Source: CAD feature listing. Evaluate the final solid. Frame: model axes, mm. Face numbers are marked on the shaded views. A direction names the side the tool comes from. Give positions to 0.01 mm unless a question says otherwise; leave off trailing zeros. Write each loop counter-clockwise with the first axis right and the second up, starting at its lowest first coordinate (ties: lowest second). Pieces come first, ordered by that corner, then holes. Notation, with made-up numbers: M 57.5,25.25 L 84.5,25.25 A18 cw 84.5,42.25 Z; hole C -6,29.5 d4. An arc over 180 degrees is marked long. Return JSON: item names as keys, results as strings.
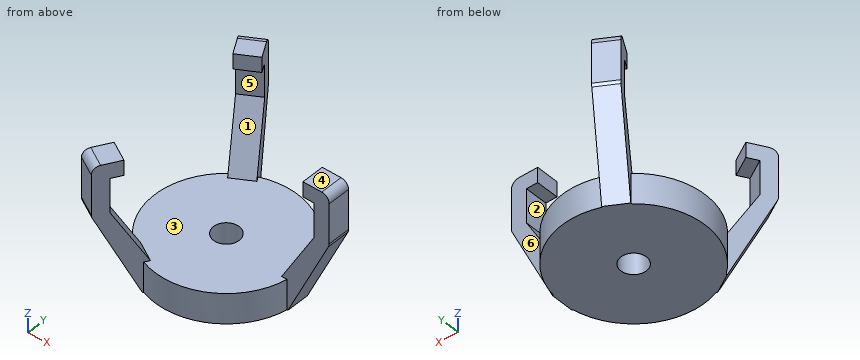
```python
from build123d import *

# Parameters (mm, degrees)
CYLINDER001_R      = 1.7
CYLINDER001_DEPTH  = 10
CYLINDER_R         = 9.5
CYLINDER_DEPTH     = 4
PAD_DEPTH          = 1.5
POLARPATTERN_COUNT = 3
FILLET_R           = 1


with BuildPart() as boltcylinder:
    # Cylinder001 → Cylinder001 (new body)
    with BuildSketch(Plane.XY):
        Circle(CYLINDER001_R)
    extrude(amount=CYLINDER001_DEPTH)


with BuildPart() as basecylinder:
    # Cylinder → Cylinder (new body)
    with BuildSketch(Plane.XY):
        Circle(CYLINDER_R)
    extrude(amount=CYLINDER_DEPTH)


with BuildPart() as fillet_body:
    # Sketch → Pad (new body, symmetric)
    with BuildSketch(Plane.XZ):
        Polygon((0, 0), (0, 2), (7.5, 2), (13, 11.5), (13, 16), (11.5, 16), (11.5, 18), (15, 18), (15, 11.5), (9.5, 0), align=None)
    pad = extrude(amount=PAD_DEPTH, both=True)

    # PolarPattern: Pad ×3 about axis
    polarpattern_axis = Axis((0, 0, 0), (0, 0, 1))
    for i in range(1, POLARPATTERN_COUNT):
        add(pad.rotate(polarpattern_axis, i * 360 / POLARPATTERN_COUNT))

    # Fusion: union BaseCylinder
    add(basecylinder.part)

    # Cut: cut BoltCylinder
    add(boltcylinder.part, mode=Mode.SUBTRACT)

    # Fillet
    fillet_edges = [fillet_body.edges().sort_by_distance(p)[0] for p in [
        (-7.5, 12.990381, 11.5),
        (-7.5, 12.990381, 18),
        (-7.5, -12.990381, 11.5),
        (15, 0, 11.5),
        (-7.5, -12.990381, 18),
        (15, 0, 18),
    ]]
    fillet(fillet_edges, radius=FILLET_R)


solid = fillet_body.part
```
1) Cut plane A-A, the plane x = 0. Return the cut outline in (y, z).
Numbers:
{"outline": "M -9.5,0 L -1.7,0 L -1.7,4 L -9.5,4 Z; M 1.7,0 L 9.5,0 L 9.5,4 L 1.7,4 Z"}
2) Cut plane D-D, the plane z = 12.75. Return the cut outline in (x, y), then the cut area to 3 significant figures.
Numbers:
{"outline": "M -8.8,-12.24 L -6.2,-13.74 L -5.2,-12.01 L -7.8,-10.51 Z; M -8.8,12.24 L -7.8,10.51 L -5.2,12.01 L -6.2,13.74 Z; M 13,-1.5 L 15,-1.5 L 15,1.5 L 13,1.5 Z", "area": "18.0 mm²"}
3) Line query: line 1 (Y direction, x = 0, z = 1.5); line 2 (Z direction, x = 6, y = 4); line 3 (Y direction, x = 11, z = 6.5). Output: solid intervals per line, ascending. Write a range as [from, to].
Numbers:
{"line 1": "y = [-9.5, -1.7], [1.7, 9.5]", "line 2": "z = [0, 4]", "line 3": "y = [-1.5, 1.5]"}
4) Contact query for flat-ended pins moving along their axis: pin 1 Ø5 at (x, z) = (11.5, 7.5) entering from -Y; pin 2 Ø3 at (y, z) = (-2.5, 13) entering from +X; pin 3 Ø7 at (x, z) = (11.5, 12.5) entering from +Y; pin 4 Ø3 at (x, y) = (-6, 10) entering from -Z. Output: stop coordinate, or through.
Numbers:
{"pin 1": "stops at y = -1.5", "pin 2": "stops at x = 15", "pin 3": "stops at y = 1.5", "pin 4": "stops at z = 1.38"}
5) Draft query along Z for the marked faces 4, 5 and 6. Return one class per face: released by +Z, released by -Z, zero draft, split by the parting line, or undercut.
Numbers:
{"face 4": "released by +Z", "face 5": "undercut", "face 6": "zero draft"}
6) Cut plane C-C, the plane z = 16.5. Return the cut outline in (x, y), then the cut area to 3 significant figures.
Numbers:
{"outline": "M -8.8,-12.24 L -6.2,-13.74 L -4.45,-10.71 L -7.05,-9.21 Z; M -8.8,12.24 L -7.05,9.21 L -4.45,10.71 L -6.2,13.74 Z; M 11.5,-1.5 L 15,-1.5 L 15,1.5 L 11.5,1.5 Z", "area": "31.5 mm²"}
7) Cut plane B-B, the plane y = 0. Return the cut outline in (x, z), then the cut area to 3 significant figures.
Numbers:
{"outline": "M -9.5,0 L -1.7,0 L -1.7,4 L -9.5,4 Z; M 1.7,0 L 9.5,0 L 14.9,11.3 A1 ccw 15,11.73 L 15,17 A1 ccw 14,18 L 11.5,18 L 11.5,16 L 13,16 L 13,11.5 L 8.66,4 L 1.7,4 Z", "area": "99.8 mm²"}
8) Set-up query: the marked faces 1, 2 and 3. Return all of +Z, -Z, +X, -X, +Y, -Y with unobstructed straight access to the full face (end or side cutting, diameter ignored); none if empty.
Numbers:
{"face 1": "+X", "face 2": "-X, +Y, -Y", "face 3": "+Z"}
